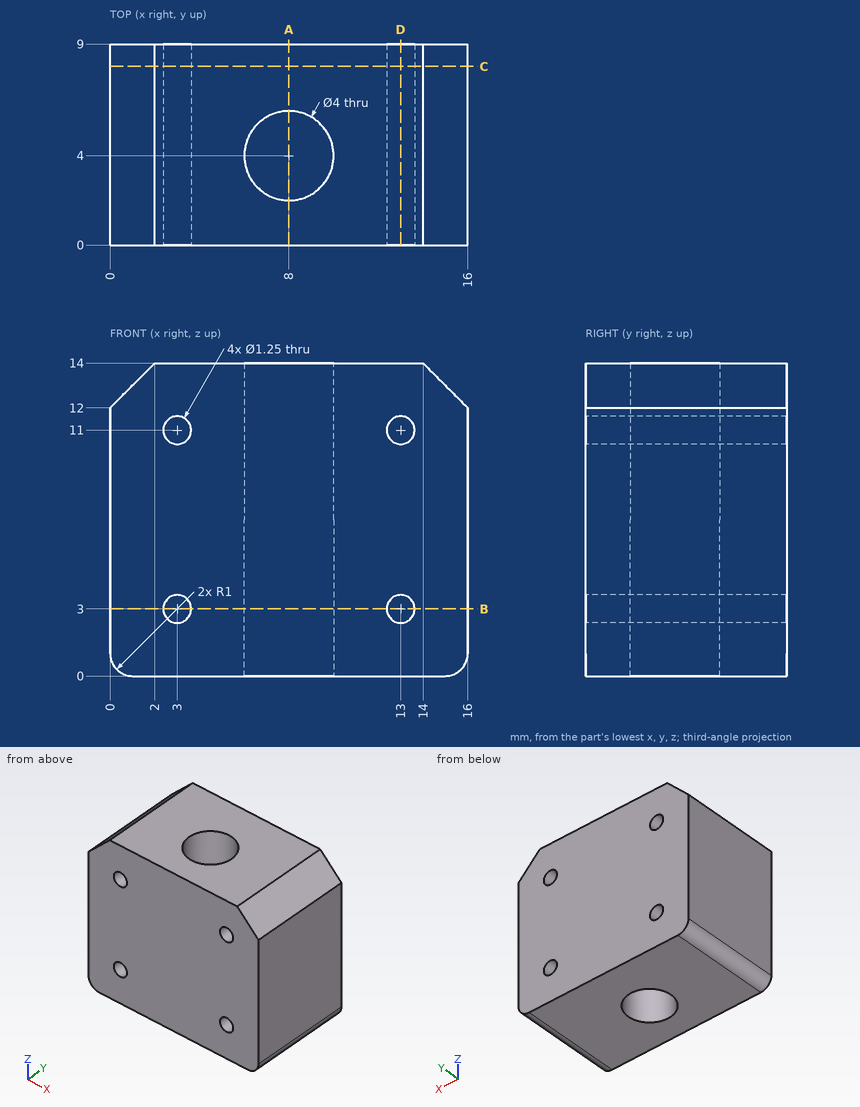
Answer from the drawing. Dimensions are ordinates in mm from the lowest x, y and z of the part. Coordinates: 2 decimals unless noted, no trailing zeros. Loops run counter-clockwise (first coordinate to the right, second up) from the corner with the lowest first, then second, coordinate; pieces in that order, holes last.
Q1. The part is cut by section D-D on x = 13. Write down the section's boundary in (y, z) (3 decimals), and give its area (4 significant figures).
Q2. The part is cut by section A-A on x = 8. Write down the section's boundary in (y, z).
Q3. The part is cut by section C-C on y = 8. Write down the section's boundary in (x, z) (3 decimals), and give its area (3 significant figures).
Q4. Consider probe 1 along X at (y, z) = (6.25, 11) (3 decimals); probe 2 along Z at (x, y) = (2.75, 2.25); probe 3 along X at (y, z) = (4.5, 11) (1 decimal). Determine where each line is inside the solid, lowest interval first.
Q5. This flat-tipped pin is pushed along its axis until it touches: pin 1 Ø0.8 at (x, z) = (13, 3) entering from -Y. Where does it stop, or does it pass through?
Q6. The part is cut by section B-B on z = 3. Write down the section's boundary in (x, y) (3 decimals), and give its area (3 significant figures).
Results below:
1. outline: (0, 0) - (9, 0) - (9, 2.375) - (0, 2.375) - close; (0, 3.625) - (9, 3.625) - (9, 10.375) - (0, 10.375) - close; (0, 11.625) - (9, 11.625) - (9, 14) - (0, 14) - close
1. area: 103.5 mm2
2. outline: (0, 0) - (2, 0) - (2, 14) - (0, 14) - close; (6, 0) - (9, 0) - (9, 14) - (6, 14) - close
3. outline: (0, 1) arc R1 ccw to (1, 0) - (15, 0) arc R1 ccw to (16, 1) - (16, 12) - (14, 14) - (2, 14) - (0, 12) - close; hole circle Ø1.25 at (3, 3); hole circle Ø1.25 at (3, 11); hole circle Ø1.25 at (13, 3); hole circle Ø1.25 at (13, 11)
3. area: 215 mm2
4. probe 1: x = 0 to 2.375, 3.625 to 12.375, 13.625 to 16
4. probe 2: z = 0 to 2.43, 3.57 to 10.43, 11.57 to 14
4. probe 3: x = 0 to 2.4, 3.6 to 6.1, 9.9 to 12.4, 13.6 to 16
5. pin 1: passes through
6. outline: (0, 0) - (2.375, 0) - (2.375, 9) - (0, 9) - close; (3.625, 0) - (12.375, 0) - (12.375, 9) - (3.625, 9) - close; (13.625, 0) - (16, 0) - (16, 9) - (13.625, 9) - close; hole circle Ø4 at (8, 4)
6. area: 109 mm2
